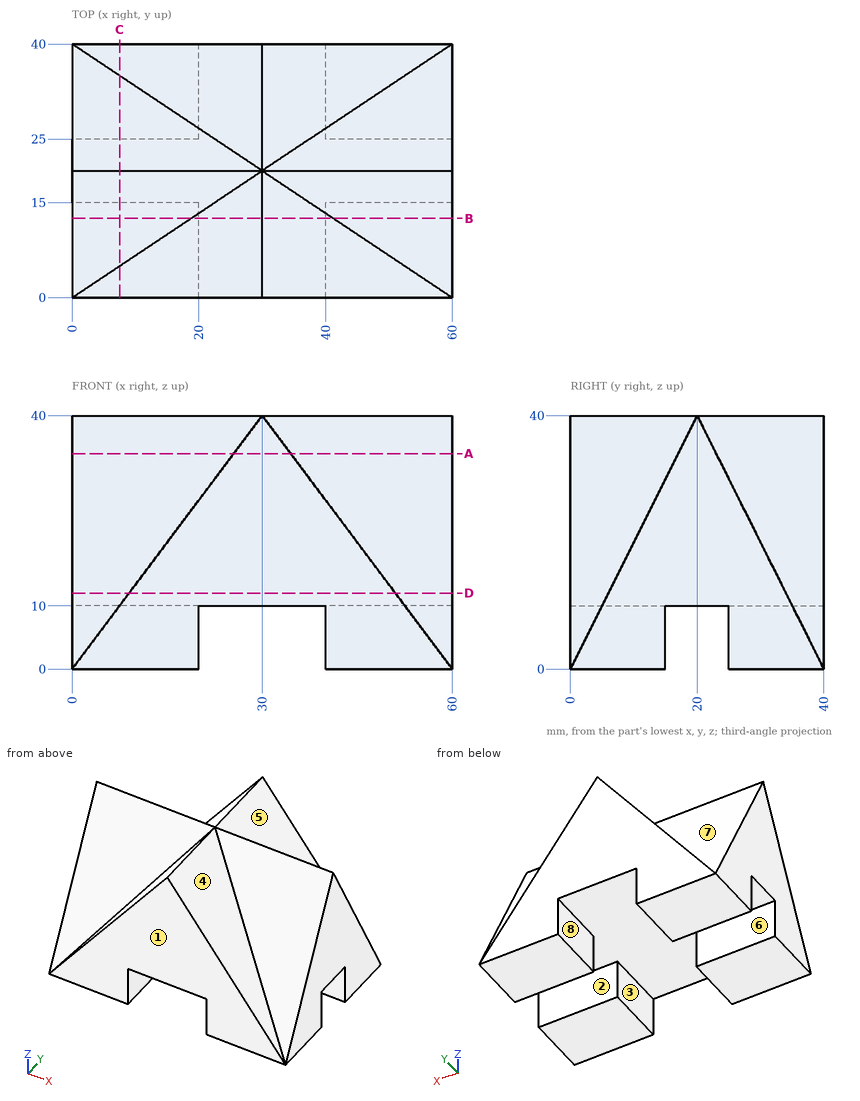
For this review, use the dimensioned drawing (mm, ordinates from the lowest corner) and the shaded views. A direction names the side the tool comes from. Round coordinates to 2 decimals unless told otherwise and drop trailing zeros. Write each loop counter-clockwise with the first axis right and the second up, starting at its lowest first coordinate (ties: lowest second). Pieces come first, ordered by that corner, then holes. Notation, with made-up numbers: (-12, 71) - (32, 71) arc R27 cw to (32, 87) - close; hole circle Ø1 at (5.25, 29). An arc over 180 degrees is marked (long way). Answer as a JSON object with one key per item and string values.
1. We need section B-B on y = 12.5. Give the boundary of the cut face in (x, z).
Response values:
{"outline": "(0, 0) - (20, 0) - (20, 10) - (40, 10) - (40, 0) - (60, 0) - (60, 25) - (41.25, 25) - (30, 40) - (18.75, 25) - (0, 25) - close"}
2. To check wall thickness, follow line 1 along Y through (x, z) = (56, 2.5); line 2 along X through (y, z) = (11.5, 2.5); line 3 along Z through (x, y) = (46.5, 36.5). State the ranges of each line that lie inside material, in increasing order.
Response values:
{"line 1": "y = 0 to 15, 25 to 40", "line 2": "x = 0 to 20, 40 to 60", "line 3": "z = 0 to 18"}
3. We need section A-A on z = 34. Give the boundary of the cut face in (x, y), then the cut area to 3 significant figures.
Response values:
{"outline": "(0, 17) - (25.5, 17) - (25.5, 0) - (34.5, 0) - (34.5, 17) - (60, 17) - (60, 23) - (34.5, 23) - (34.5, 40) - (25.5, 40) - (25.5, 23) - (0, 23) - close", "area": "666 mm2"}
4. For pin 1 Ø5 at (y, z) = (7, 30) entering from -X (3 decimals); pin 2 Ø1.5 at (x, y) = (23.5, 10.5) entering from +Z, all flat-tipped, find the tip position at first contact; note any pin that passes through.
Response values:
{"pin 1": "stops at x = 20.625", "pin 2": "stops at z = 32.33"}
5. Draft analysis for pull direction Y (two halves, no side actions). For the marked faces 1, 2 and 3, state which applies: +Y half, -Y half, draft (parallel to the pull), parting line (faces both ways), or undercut.
Response values:
{"face 1": "-Y half", "face 2": "undercut", "face 3": "draft"}
6. We need section D-D on z = 12. Give the boundary of the cut face in (x, y).
Response values:
{"outline": "(0, 6) - (9, 6) - (9, 0) - (51, 0) - (51, 6) - (60, 6) - (60, 34) - (51, 34) - (51, 40) - (9, 40) - (9, 34) - (0, 34) - close"}
7. We need section C-C on x = 7.5. Give the boundary of the cut face in (y, z), then the cut area to 3 significant figures.
Response values:
{"outline": "(0, 0) - (15, 0) - (15, 10) - (25, 10) - (25, 0) - (40, 0) - (40, 10) - (35, 10) - (20, 40) - (5, 10) - (0, 10) - close", "area": "750 mm2"}
8. Tool access review of the marked faces 4, 5, 6, 7 and 8: name each direction out of +Z, -Z, +X, -X, +Y, -Y from which nothing blocks a thin tool from reaching the whole face with its end or side.
Response values:
{"face 4": "+Z, +X, -Y", "face 5": "+Z, +X, +Y", "face 6": "-Z, +X, -X", "face 7": "+Z, -X, +Y", "face 8": "-Z, +Y, -Y"}
